from build123d import *

# Parameters (mm, degrees)
F0_R     = 14.4
F1_DEPTH = 8
F0_R_2   = 0.5
F2_DEPTH = 24
F4_DEPTH = 25
F5_R     = 14.4
F6_DEPTH = 1


# Not quite as in the source:
# - a feature names something its author has since deleted; it is built from what else it names


with BuildPart() as f1:
    # F0 (on Front) → F1 (new body)
    with BuildSketch(Plane.XZ):
        with Locations((0.0303304768, -0.0397499959)):
            Circle(F0_R)
        with BuildLine():
            ThreePointArc((10.6755009314, 7.8496635433), (12.4816793636, 4.6139026446), (13.301518859, 1))
            ThreePointArc((13.301518859, 1), (13.3431044371, 0.0001181292), (13.3076524455, -1))
            ThreePointArc((13.3076524455, -1), (12.4958940048, -4.6561546149), (10.6755009314, -7.9291635352))
            ThreePointArc((10.6755009314, -7.9291635352), (-3.6648740835, -12.7640559989), (-13.1848282407, -1))
            ThreePointArc((-13.1848282407, -1), (-13.2196095565, 0.0001136945), (-13.1788110527, 1))
            ThreePointArc((-13.1788110527, 1), (-11.605380035, 6.2984469785), (-8.0072458781, 10.4939989255))
            ThreePointArc((-8.0072458781, 10.4939989255), (-7.1861367371, 11.0726350293), (-6.3235511773, 11.5874030488))
            ThreePointArc((-6.3235511773, 11.5874030488), (2.8757590992, 12.9011168976), (10.6755009314, 7.8496635433))
        make_face(mode=Mode.SUBTRACT)
    extrude(amount=F1_DEPTH)

    # F0 (on Front) → F2 (join)
    with BuildSketch(Plane.XZ):
        with Locations((0.0303304768, -0.0397499959)):
            Circle(F0_R)
        with BuildLine():
            ThreePointArc((10.6755009314, 7.8496635433), (12.4816793636, 4.6139026446), (13.301518859, 1))
            ThreePointArc((13.301518859, 1), (13.3431044371, 0.0001181292), (13.3076524455, -1))
            ThreePointArc((13.3076524455, -1), (12.4958940048, -4.6561546149), (10.6755009314, -7.9291635352))
            ThreePointArc((10.6755009314, -7.9291635352), (-3.6648740835, -12.7640559989), (-13.1848282407, -1))
            ThreePointArc((-13.1848282407, -1), (-13.2196095565, 0.0001136945), (-13.1788110527, 1))
            ThreePointArc((-13.1788110527, 1), (-11.605380035, 6.2984469785), (-8.0072458781, 10.4939989255))
            ThreePointArc((-8.0072458781, 10.4939989255), (-7.1861367371, 11.0726350293), (-6.3235511773, 11.5874030488))
            ThreePointArc((-6.3235511773, 11.5874030488), (2.8757590992, 12.9011168976), (10.6755009314, 7.8496635433))
        make_face(mode=Mode.SUBTRACT)
        with BuildLine():
            ThreePointArc((11.3320508076, -1), (11.5318516526, -0.5176380902), (11.6, 0))
            ThreePointArc((11.6, 0), (11.5318516526, 0.5176380902), (11.3320508076, 1))
            ThreePointArc((11.3320508076, 1), (7.6, 0), (11.3320508076, -1))
        make_face()
        with Locations((9.6801056635, 0)):
            Circle(F0_R_2, mode=Mode.SUBTRACT)
        with BuildLine():
            ThreePointArc((-10.2180339887, 1), (-10.6, 0), (-10.2180339887, -1))
            ThreePointArc((-10.2180339887, -1), (-8.5647668653, -1.4012585384), (-7.6, 0))
            ThreePointArc((-7.6, 0), (-8.5647668653, 1.4012585384), (-10.2180339887, 1))
        make_face()
        with Locations((-9.119440236, 0)):
            Circle(F0_R_2, mode=Mode.SUBTRACT)
        with BuildLine():
            ThreePointArc((-3.7285347361, 8.0512374523), (-4.0895399111, 9.0272962561), (-4.9987891209, 9.5335386876))
            ThreePointArc((-4.9987891209, 9.5335386876), (-6.0454932887, 9.3092433042), (-6.6761302568, 8.4442606176))
            ThreePointArc((-6.6761302568, 8.4442606176), (-5.4267854851, 6.5643962904), (-3.7285347361, 8.0512374523))
        make_face()
        with Locations((-5.2285347361, 8.0512374523)):
            Circle(F0_R_2, mode=Mode.SUBTRACT)
        with BuildLine():
            ThreePointArc((-13.1788110527, 1), (-13.2196095565, 0.0001136945), (-13.1848282407, -1))
            Line((-13.1848282407, -1), (-10.8320508076, -1))
            Line((-10.8320508076, -1), (-10.2180339887, -1))
            ThreePointArc((-10.2180339887, -1), (-10.6, 0), (-10.2180339887, 1))
            Line((-10.2180339887, 1), (-10.8320508076, 1))
            Line((-10.8320508076, 1), (-13.1788110527, 1))
        make_face()
        with BuildLine():
            Line((-4.9987891209, 9.5335386876), (-6.3235511773, 11.5874030488))
            ThreePointArc((-6.3235511773, 11.5874030488), (-7.1861367371, 11.0726350293), (-8.0072458781, 10.4939989255))
            Line((-8.0072458781, 10.4939989255), (-6.6761302568, 8.4442606176))
            ThreePointArc((-6.6761302568, 8.4442606176), (-6.0454932887, 9.3092433042), (-4.9987891209, 9.5335386876))
        make_face()
        with BuildLine():
            ThreePointArc((11.3320508076, 1), (11.5318516526, 0.5176380902), (11.6, 0))
            ThreePointArc((11.6, 0), (11.5318516526, -0.5176380902), (11.3320508076, -1))
            Line((11.3320508076, -1), (13.25, -1))
            Line((13.25, -1), (13.3076524455, -1))
            ThreePointArc((13.3076524455, -1), (13.3431044371, 0.0001181292), (13.301518859, 1))
            Line((13.301518859, 1), (13.25, 1))
            Line((13.25, 1), (11.3320508076, 1))
        make_face()
    extrude(amount=-F2_DEPTH)

    # F3 (on Top) → F4 (cut)
    with BuildSketch(Plane.XY):
        with BuildLine():
            Line((1.6, 6.2556717858), (1.6, 8.2034006216))
            ThreePointArc((1.6, 8.2034006216), (0, 7.5556717858), (-1.6, 8.2034006216))
            Line((-1.6, 8.2034006216), (-1.6, 6.2556717858))
            Line((-1.6, 6.2556717858), (1.6, 6.2556717858))
        make_face()
        with BuildLine():
            ThreePointArc((1.6, 8.2034006216), (2.1177818585, 8.9584538635), (2.3, 9.8556717858))
            ThreePointArc((2.3, 9.8556717858), (2.1177818585, 10.752889708), (1.6, 11.50794295))
            ThreePointArc((1.6, 11.50794295), (0, 12.1556717858), (-1.6, 11.50794295))
            ThreePointArc((-1.6, 11.50794295), (-2.3, 9.8556717858), (-1.6, 8.2034006216))
            ThreePointArc((-1.6, 8.2034006216), (0, 7.5556717858), (1.6, 8.2034006216))
        make_face()
        with BuildLine():
            ThreePointArc((-1.6, 11.50794295), (0, 12.1556717858), (1.6, 11.50794295))
            Line((1.6, 11.50794295), (1.6, 13.4556717858))
            Line((1.6, 13.4556717858), (-1.6, 13.4556717858))
            Line((-1.6, 13.4556717858), (-1.6, 11.50794295))
        make_face()
    extrude(amount=F4_DEPTH, mode=Mode.SUBTRACT)

    # F5 (on face) → F6 (join)
    with BuildSketch(Plane(origin=(0, 24, 0), x_dir=(-1, 0, 0), z_dir=(0, 1, 0))):
        Circle(F5_R)
    extrude(amount=F6_DEPTH)


solid = f1.part
The listing builds one solid part. Answer for the finished solid, in the listing's coordinates (mm). A direction names the side the tool comes from. Coordinates: 2 decimals unless noted, no trailing zeros. Write each loop counter-clockwise with the first axis right and the second up, starting at its lowest first coordinate (ties: lowest second). Pieces come first, ordered by that corner, then holes. Notation, with made-up numbers: M 49,18.5 L 68,18.5 A16 ccw 68,28.5 Z; hole C 83.25,71 d5. An arc over 180 degrees is marked long. Use one line per item in the form item = value.
Item 1: The mould has two halves that part along X. Classify faces 1 (the face through (-5, 24, 8)), 2 (the face through (-13.735, 24.493, 4.325)), 3 (the face through (13, -8, -4)): released by +X, released by -X, zero draft, split by the parting line, or undercut.
Model answer:
face_1 = undercut
face_2 = split by the parting line
face_3 = zero draft
Item 2: Find section C-C, the plane y = -0.5. Give the vertices of the cut face in (x, z), plus the area to 3 significant figures.
Model answer:
outline = C 0.03,-0.04 d28.8; hole M 10.68,-7.93 A13 ccw 10.68,7.85 A13.25 ccw long Z
area = 99.2 mm2
Item 3: Find section B-B, the plane y = 20.5. Give the vertices of the cut face in (x, z), plus the area to 3 significant figures.
Model answer:
outline = C 0.03,-0.04 d28.8; hole M -13.18,-1 A13.25 ccw 10.68,-7.93 A13 ccw 13.31,-1 L 11.33,-1 A2 cw long 11.33,1 L 13.3,1 A13 ccw 10.68,7.85 A13.25 ccw -6.32,11.59 L -5,9.53 A1.5 cw long -6.68,8.44 L -8.01,10.49 A13.25 ccw -13.18,1 L -10.22,1 A1.5 cw long -10.22,-1 Z; hole C -9.12,0 d1; hole C -5.23,8.05 d1; hole C 9.68,0 d1
area = 137 mm2
Item 4: Given P1, Ø5, axis at x = -0.5, y = 7, coming from the +Z side; P2, Ø3.5, axis at x = -5, z = 10.5, coming from the -Y side; P3, Ø1.1, axis at x = -9.5, z = 0, coming from the -Y side; P4, Ø6, axis at x = 0, z = -8, coming from the -Y side, each flat-ended and moving along its own axis, determine where each tip first touches the part or whether it passes through.
Model answer:
P1 = 14.36
P2 = -8
P3 = 0
P4 = 24
Item 5: For faces 4 (the face through (0, 25, 0)), 5 (the face through (1.6, 12, 14)), 6 (the face through (0, 24, 0)), determine the directions among +Z, -Z, +X, -X, +Y, -Y from which every point of the face is accessible in a straight line to the end or side of a thin tool.
Model answer:
face_4 = +Z, -Z, +X, -X, +Y
face_5 = +Z
face_6 = -Y
Item 6: Find the intervals of material crossed by probe 1 along Z at (x, y) = (11, 7) (1 decimal); probe 2 along Z at (x, y) = (10, 13); probe 3 along Z at (x, y) = (-5.5, 1), in increasing order.
Model answer:
probe_1 = -9.4 to -7.5, -1.4 to 1.4, 7.4 to 9.3
probe_2 = -10.43 to -8.77, -1.96 to -0.38, 0.38 to 1.96, 8.69 to 10.35
probe_3 = -13.34 to -12.08, 6.58 to 7.63, 8.47 to 10.31, 12 to 13.26
